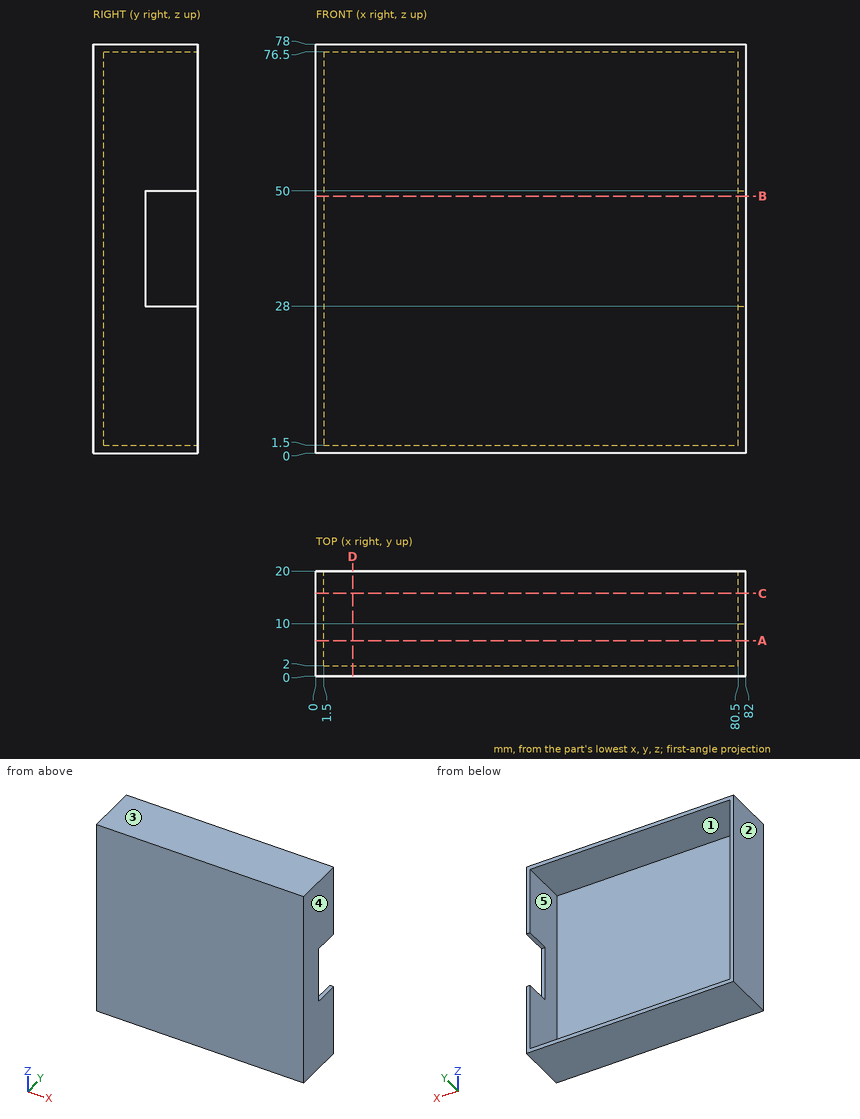
Verification items for this drawing (mm, ordinates from the low corner). A direction names the side the tool comes from. Coordinates: 2 decimals unless noted, no trailing zeros. Write each loop counter-clockwise with the first axis right and the second up, starting at its lowest first coordinate (ties: lowest second). Pieces come first, ordered by that corner, then holes. Notation, with made-up numbers: M 6.5,36 L 12.5,36 A10 ccw 12.5,55 Z; hole C 14.25,21 d3. An arc over 180 degrees is marked long. Answer as a JSON object with one key per item and string values. Group by question number.
(1) Cross-section at B-B, the plane z = 49. Record the cut outline in (x, y).
(2) Tool access check on the marked faces 4 and 5. Record the directions out of +Z, -Z, +X, -X, +Y, -Y that give a thin tool (end or side, any length) a straight path to the whole face; none if there is none.
(3) Gauge pin test, flat ends, axial feed: pin 1 (1.5 mm diameter, centred on x = 69.5, z = 11.5, fed in from +Y); pin 2 (4 mm diameter, centred on x = 27, y = 3, fed in from -Z); pin 3 (1.2 mm diameter, centred on x = 81, z = 42.5, fed in from +Y). Record the tip position at first contact, or that the pin passes through.
(4) Cross-section at A-A, the plane y = 6.75. Record the cut outline in (x, z).
(5) Release check for a two-part mould opening along Z. For the marked faces 1, 2 and 3 record: +Z half, -Z half, draft (parallel to the pull), parting line (faces both ways), or undercut.
(6) Cross-section at D-D, the plane x = 7. Record the cut outline in (y, z).
(7) Material ranges on line 1 (Z direction, x = 68, y = 14); line 2 (X direction, y = 6.5, z = 18); line 3 (Y direction, x = 19, z = 41), recorded low to high.
(8) Cross-section at C-C, the plane y = 15.75. Record the cut outline in (x, z).
Reply:
{
 "1": {"outline": "M 0,0 L 82,0 L 82,10 L 80.5,10 L 80.5,2 L 1.5,2 L 1.5,20 L 0,20 Z"},
 "2": {"face 4": "+Z, -Z, +X, +Y, -Y", "face 5": "+Y"},
 "3": {"pin 1": "y = 2", "pin 2": "z = 0", "pin 3": "y = 10"},
 "4": {"outline": "M 0,0 L 82,0 L 82,78 L 0,78 Z; hole M 1.5,1.5 L 80.5,1.5 L 80.5,76.5 L 1.5,76.5 Z"},
 "5": {"face 1": "undercut", "face 2": "draft", "face 3": "+Z half"},
 "6": {"outline": "M 0,0 L 20,0 L 20,1.5 L 2,1.5 L 2,76.5 L 20,76.5 L 20,78 L 0,78 Z"},
 "7": {"line 1": "0 to 1.5, 76.5 to 78", "line 2": "0 to 1.5, 80.5 to 82", "line 3": "0 to 2"},
 "8": {"outline": "M 0,0 L 82,0 L 82,28 L 80.5,28 L 80.5,1.5 L 1.5,1.5 L 1.5,76.5 L 80.5,76.5 L 80.5,50 L 82,50 L 82,78 L 0,78 Z"}
}
